Can you work these out from the model? Positions are in its coordinate system, mm. Face numbers are marked on the shaded views. A direction names the side the tool comes from. Coordinates: 2 decimals unless noted, no trailing zeros. Order: outer loops, then holes, each group sorted by start corner. A loop starts at its lowest first (then second) coordinate and runs counter-clockwise, first axis right, second up. Notation, with made-up numbers: (40.25, 68) -> (58.25, 68) arc R15 ccw to (58.25, 84) -> close; hole circle Ø10 at (44, -25). An arc over 180 degrees is marked (long way). Answer in a Markdown table with one row per item. Add a question column.
1. Will these pins go through, and if not, where does the flat tip stop? pin 1 (1.5 mm diameter, centred on x = -9, z = 15, fed in from -Y); pin 2 (10 mm diameter, centred on x = -6.5, z = 14, fed in from +Y); pin 3 (7 mm diameter, centred on x = 23, y = -19, fed in from +Z).
2. We'd pull the mould along Y, two halves only. Please class the marked faces 5, 6, 7 and 8: pulls with the +Y half, pulls with the -Y half, needs draft (parallel to the pull), parting line crosses it, or undercut.
3. On a 3-axis mill with a long thin cutter (end or side, diameter ignored), from which of +Z, -Z, +X, -X, +Y, -Y can I reach the whole of each face in a straight line? I mean the marked faces 1, 2, 3 and 4. Say none if no direction works.
4. Imagine slicing it at D-D on x = 23. Write out the boundary of the cut face in (y, z) (3 decimals).
5. Imagine slicing it at A-A on z = 8.75. Write out the boundary of the cut face in (x, y), plus the area to 3 significant figures.
6. Imagine slicing it at C-C on y = -28. Write out the boundary of the cut face in (x, z).
7. If I drill on line 1 along Y through (x, z) = (-23, 0.5); line 2 along Y through (x, z) = (-23, 13) (3 decimals); line 3 along Z through (x, y) = (10, -26.5), over which ranges is the centre line in solid material (lowest first)? Write a range as [from, to].
8. Imagine slicing it at B-B on y = -21. Write out the boundary of the cut face in (x, z), plus the area to 3 significant figures.
from build123d import *

# Parameters (mm, degrees)
F0_R           = 14
F0_R_2         = 6
F1_DEPTH       = 25
F3_D           = 6.3
F3_CBORE_D     = 11.25
F3_CBORE_DEPTH = 6
F4_SIZE        = 2.5
F5_W           = 34
F5_H           = 36
F5_R           = 6
F6_DEPTH       = 5
F7_SIZE        = 2.49999
F8_R           = 6
F9_DEPTH       = 4
F10_SIZE       = 3
F11_DEPTH      = 5


# Not quite as in the source:
# - a fillet or chamfer is up to 0.001 mm smaller than in the source, because OpenCascade refuses the exact size
# - a feature names something its author has since deleted; it is built from what else it names


with BuildPart() as f1:
    # F0 (on Front) → F1 (new body)
    with BuildSketch(Plane.XZ):
        Polygon((-30, 16.25), (-30, -16.25), (30, -16.25), (30, 16.25), (17, 16.25), (17, 26.75), (-17, 26.75), (-17, 16.25), align=None)
        with Locations((0, 8.75)):
            Circle(F0_R, mode=Mode.SUBTRACT)
        with Locations((0, 8.75)):
            Circle(F0_R)
        with Locations((0, 8.75)):
            Circle(F0_R_2, mode=Mode.SUBTRACT)
    extrude(amount=F1_DEPTH)

    # F3 (through all)
    with Locations(Plane.XY.offset(16.25)):
        with Locations((-23, -6), (-23, -19), (23, -6), (23, -19)):
            CounterBoreHole(F3_D / 2, F3_CBORE_D / 2, F3_CBORE_DEPTH)

    # F4
    f4_edges = [f1.edges().sort_by_distance(p)[0] for p in [
        (17, -12.5, 26.75),
        (-17, -12.5, 26.75),
    ]]
    chamfer(f4_edges, length=F4_SIZE)

    # F5 (on face) → F6 (join)
    with BuildSketch(Plane.XZ.offset(25)):
        with Locations((0, 8.75)):
            Rectangle(F5_W, F5_H)
        with Locations((0, 8.75)):
            Circle(F5_R, mode=Mode.SUBTRACT)
    extrude(amount=F6_DEPTH)

    # F7 (size 2.5 in the source; OpenCascade refuses exactly that, so slightly less here)
    f7_edges = [f1.edges().sort_by_distance(p)[0] for p in [
        (17, -27.5, 26.75),
        (-17, -27.5, 26.75),
        (17, -27.5, -9.25),
        (-17, -27.5, -9.25),
    ]]
    chamfer(f7_edges, length=F7_SIZE)

    # F8 (on face) → F9 (join)
    with BuildSketch(Plane.XZ.offset(30)):
        Polygon((0, 21.4779220614), (-12.7279220614, 8.75), (0, -3.9779220614), (12.7279220614, 8.75), align=None)
        with Locations((0, 8.75)):
            Circle(F8_R, mode=Mode.SUBTRACT)
    extrude(amount=F9_DEPTH)

    # F10
    f10_edges = [f1.edges().sort_by_distance(p)[0] for p in [
        (0, -32, 21.477922),
        (12.727922, -32, 8.75),
        (-12.727922, -32, 8.75),
        (0, -32, -3.977922),
    ]]
    chamfer(f10_edges, length=F10_SIZE)

    # F0 (on Front) → F11 (cut)
    with BuildSketch(Plane.XZ):
        with Locations((0, 8.75)):
            Circle(F0_R)
        with Locations((0, 8.75)):
            Circle(F0_R_2, mode=Mode.SUBTRACT)
    extrude(amount=F11_DEPTH, mode=Mode.SUBTRACT)


solid = f1.part
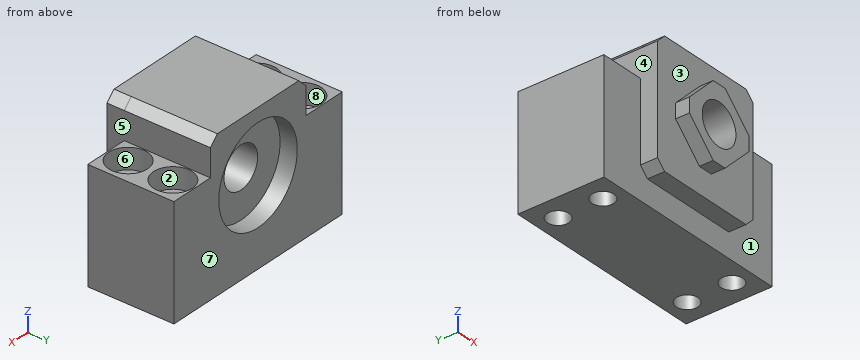
Answers follow:
| question | item | result |
|---|---|---|
| 1 | pin 1 | stops at y = -30 |
| 1 | pin 2 | stops at y = -5 |
| 1 | pin 3 | stops at z = 10.25 |
| 2 | face 5 | needs draft |
| 2 | face 6 | undercut |
| 2 | face 7 | pulls with the +Y half |
| 2 | face 8 | undercut |
| 3 | face 1 | -Z, -Y |
| 3 | face 2 | +Z |
| 3 | face 3 | -Y |
| 3 | face 4 | +Z, -X, -Y |
| 4 | outline | (-25, -16.25) -> (-22.15, -16.25) -> (-22.15, 10.25) -> (-24.625, 10.25) -> (-24.625, 16.25) -> (-25, 16.25) -> close; (-15.85, -16.25) -> (-9.15, -16.25) -> (-9.15, 10.25) -> (-11.625, 10.25) -> (-11.625, 16.25) -> (-13.375, 16.25) -> (-13.375, 10.25) -> (-15.85, 10.25) -> close; (-2.85, -16.25) -> (0, -16.25) -> (0, 16.25) -> (-0.375, 16.25) -> (-0.375, 10.25) -> (-2.85, 10.25) -> close |
| 5 | outline | (-30, -25) -> (-17, -25) -> (-17, -30) -> (-10.61, -30) -> (-10.61, -34) -> (-6, -34) -> (-6, -5) -> (-14, -5) -> (-14, 0) -> (-30, 0) -> close; (6, -34) -> (10.61, -34) -> (10.61, -30) -> (17, -30) -> (17, -25) -> (30, -25) -> (30, 0) -> (14, 0) -> (14, -5) -> (6, -5) -> close; hole circle Ø6.3 at (-23, -19); hole circle Ø6.3 at (-23, -6); hole circle Ø6.3 at (23, -19); hole circle Ø6.3 at (23, -6) |
| 5 | area | 1,140 mm² |
| 6 | outline | (-17, -6.75) -> (-14.5, -9.25) -> (14.5, -9.25) -> (17, -6.75) -> (17, 24.25) -> (14.5, 26.75) -> (-14.5, 26.75) -> (-17, 24.25) -> close; hole circle Ø12 at (0, 8.75) |
| 7 | line 1 | y = [-25, -22.15], [-15.85, -9.15], [-2.85, 0] |
| 7 | line 2 | y = [-25, -24.625], [-13.375, -11.625], [-0.375, 0] |
| 7 | line 3 | z = [-9.25, 26.75] |
| 8 | outline | (-30, -16.25) -> (-25.43, -16.25) -> (-25.43, 10.25) -> (-28.26, 10.25) -> (-28.26, 16.25) -> (-30, 16.25) -> close; (-20.57, -16.25) -> (20.57, -16.25) -> (20.57, 10.25) -> (17.74, 10.25) -> (17.74, 16.25) -> (17, 16.25) -> (17, 24.25) -> (14.5, 26.75) -> (-14.5, 26.75) -> (-17, 24.25) -> (-17, 16.25) -> (-17.74, 16.25) -> (-17.74, 10.25) -> (-20.57, 10.25) -> close; (25.43, -16.25) -> (30, -16.25) -> (30, 16.25) -> (28.26, 16.25) -> (28.26, 10.25) -> (25.43, 10.25) -> close; hole circle Ø12 at (0, 8.75) |
| 8 | area | 1,800 mm² |
